Source: CAD feature listing. Evaluate the final solid. Frame: model axes, mm. A direction names the side the tool comes from. Coordinates: 2 decimals unless noted, no trailing zeros. Loops run counter-clockwise (first coordinate to the right, second up) from the corner with the lowest first, then second, coordinate; pieces in that order, holes last. Notation, with made-up numbers: M 35,57.5 L 60,57.5 A24 cw 60,79.5 Z; hole C 20,64.25 d7. An arc over 180 degrees is marked long. One line per question, with ' | ' between items. Start each with the question number.
1. Ray query, probe 1 along Y at (x, z) = (0, 7.5); probe 2 along Y at (x, z) = (-2, 8.75); probe 3 along Z at (x, y) = (-12, -20). Return the intervals inside material, ascending.
2. Pin query (flat end, axial travel): P1, Ø6, axis at x = 15.5, z = 8.5, coming from the -Y side; P2, Ø1, axis at x = 17.5, y = -15.5, coming from the +Z side; P3, Ø3, axis at x = 0, y = 0, coming from the -Z side; P4, Ø2, axis at y = -17.5, z = 8.5, coming from the +X side. Return the tip coordinate at first contact, or that it passes through.
3. Mould query, pull axis X, two halves, no side actions, for faces 1 (the cylindrical face through (-1.617, -0.67, 4.93)), 2 (the flat face through (-5, 34, 10)), 3 (the cylindrical face through (-28, -21, 5)). Classes: pulls with the +X half, pulls with the -X half, needs draft (parallel to the pull), parting line crosses it, or undercut.
4. Section query D-D, the plane y = -11.5. Output: boundary loops of the cut face in (x, z).
5. Section query A-A, the plane y = 0. Output: boundary loops of the cut face in (x, z).
6. Section query C-C, the plane z = 9. Output: boundary loops of the cut face in (x, y).
7. Access query for faces 4 (the flat face through (0, -7, 0)), 5 (the cylindrical face through (18.28, 28.67, 6.06)). Directions: +Z, -Z, +X, -X, +Y, -Y. A direction counts if a zero-diameter tool reaches every point of the face in a straight line with its end or side. Return the directions, or none.
```python
from build123d import *

# Parameters (mm, degrees)
F0_R     = 35
F1_DEPTH = 10
F2_R     = 34
F3_DEPTH = 8
F4_R     = 3
F5_DEPTH = 8
F7_D     = 3.5


with BuildPart() as f1:
    # F0 (on Top) → F1 (new body)
    with BuildSketch(Plane.XY):
        Circle(F0_R)
    extrude(amount=F1_DEPTH)

    # F2 (on face) → F3 (cut)
    with BuildSketch(Plane.XY.offset(10)):
        Circle(F2_R)
    extrude(amount=-F3_DEPTH, mode=Mode.SUBTRACT)

    # F4 (on face) → F5 (join)
    with BuildSketch(Plane.XY.offset(2)):
        Circle(F4_R)
    extrude(amount=F5_DEPTH)

    # F7 (through all)
    with Locations(Plane.XY.offset(10)):
        with Locations((0, 0)):
            Hole(F7_D / 2)


solid = f1.part
```
Taken from the geometry:
1) probe 1: -35 to -34, -3 to -1.75, 1.75 to 3, 34 to 35 | probe 2: -34.94 to -33.94, -2.24 to 2.24, 33.94 to 34.94 | probe 3: 0 to 2
2) P1: y = -32.69 | P2: z = 2 | P3: through | P4: x = 30.87
3) face 1: undercut | face 2: needs draft | face 3: parting line crosses it
4) outline: M -33.06,0 L 33.06,0 L 33.06,10 L 32,10 L 32,2 L -32,2 L -32,10 L -33.06,10 Z
5) outline: M -35,0 L -1.75,0 L -1.75,10 L -3,10 L -3,2 L -34,2 L -34,10 L -35,10 Z; M 1.75,0 L 35,0 L 35,10 L 34,10 L 34,2 L 3,2 L 3,10 L 1.75,10 Z
6) outline: C 0,0 d70; C 0,0 d6; hole C 0,0 d68; hole C 0,0 d3.5
7) face 4: -Z, +X, -X, +Y, -Y | face 5: +Z
